```python
from build123d import *

# Parameters (mm, degrees)
SKETCH10_W         = 3
SKETCH10_H         = 3
HANDLE_DEPTH       = 8
SKETCH13_R         = 3
GUARD_DEPTH        = 1.5
SKETCH11_R         = 2
BLADE_DEPTH        = 25
BLADE_TAPER        = 1
BLADE_TIP_ANGLE    = 180
EASY_HAND_INSERT_R = 0.5
SCALE1_SCALE       = 2


with BuildPart() as part:
    # Sketch10 → Handle (new body)
    with BuildSketch(Plane(origin=(0, 0, 0), x_dir=(1, 0, 0), z_dir=(0, 1, 0))):
        Rectangle(SKETCH10_W, SKETCH10_H)
    extrude(amount=HANDLE_DEPTH)

    # Sketch13 → Guard (add)
    with BuildSketch(Plane(origin=(0, 8, 0), x_dir=(1, 0, 0), z_dir=(0, 1, 0))):
        with Locations(Location((0, 0, 0), (0, 0, 270))):
            Circle(SKETCH13_R)
    extrude(amount=GUARD_DEPTH)

    # Sketch11 → Blade (add)
    with BuildSketch(Plane(origin=(0, 9.5, 0), x_dir=(1, 0, 0), z_dir=(0, 1, 0))):
        Circle(SKETCH11_R)
    extrude(amount=BLADE_DEPTH, taper=BLADE_TAPER)

    # Sketch12 → Blade tip (revolve)
    with BuildSketch(Plane(origin=(0, 34.5, 0), x_dir=(1, 0, 0), z_dir=(0, 1, 0))):
        with BuildLine():
            Line((0, -1.563623377), (0, 1.563623377))
            ThreePointArc((0, 1.563623377), (-1.563623377, 0), (0, -1.563623377))
        make_face()
    revolve(axis=Axis((0, 34.5, 0), (0, 0, -1)), revolution_arc=BLADE_TIP_ANGLE)

    # Easy hand insert
    easy_hand_insert_edges = [part.edges().sort_by_distance(p)[0] for p in [
        (0, 0, 1.5),
        (-1.5, 0, 0),
        (0, 0, -1.5),
        (1.5, 0, 0),
        (1.5, 4, 1.5),
        (-1.5, 4, 1.5),
        (-1.5, 4, -1.5),
        (1.5, 4, -1.5),
    ]]
    fillet(easy_hand_insert_edges, radius=EASY_HAND_INSERT_R)


with BuildPart() as part_1:
    # Scale1: scaled about (0, 16.701239366, 0)
    add(part.part.scale(SCALE1_SCALE).moved(Location((0, -16.701239366, 0))))


solid = part_1.part
```
Check sheet for the modelled part. Datum: model origin and axes. Units: mm. A direction names the side the tool comes from. Round coordinates to 2 decimals unless told otherwise and drop trailing zeros. Order: outer loops, then holes, each group sorted by start corner. A loop starts at its lowest first (then second) coordinate and runs counter-clockwise, first axis right, second up. Notation, with made-up numbers: (63.5, 50) -> (112.5, 50) arc R25 ccw to (112.5, 65) -> close; hole circle Ø9 at (-1, 84). An arc over 180 degrees is marked (long way). Use CSV: the item, a comma, the result in double quotes.
(1) Cross-section at A-A (y = -8). Record the boundary of the cut face in (x, z), and give its area (3 significant figures).
Worked out:
outline,"(-3, -2) arc R1 ccw to (-2, -3) -> (2, -3) arc R1 ccw to (3, -2) -> (3, 2) arc R1 ccw to (2, 3) -> (-2, 3) arc R1 ccw to (-3, 2) -> close"
area,"35.1 mm²"
(2) Depth check by flat-ended pin: pin 1 (4.5 mm diameter, centred on y = -9.5, z = 1, fed in from -X); pin 2 (6 mm diameter, centred on x = 0, z = -4, fed in from +Y); pin 3 (4 mm diameter, centred on x = -4, y = 30, fed in from -Z). Enter the tip coordinate at first touch or a pass-through.
Worked out:
pin 1,"x = -3"
pin 2,"y = 55.26"
pin 3,"z = -2.89"
(3) Cross-section at C-C (y = 26.5). Record the boundary of the cut face in (x, z), and give its area (3 significant figures).
Worked out:
outline,"circle Ø7.16 at (0, 0)"
area,"40.2 mm²"
(4) Tool access check on faces 1 (the face through (-0.771, 27.649, 3.473)), 2 (the face through (-3, -8, 0)), 3 (the face through (0, -8, -3)). Record the directions out of +Z, -Z, +X, -X, +Y, -Y that give a thin tool (end or side, any length) a straight path to the whole face; none if there is none.
Worked out:
face 1,"+Y"
face 2,"+Z, -Z, -X, -Y"
face 3,"-Z, +X, -X, -Y"
(5) Cross-section at B-B (y = 49). Record the boundary of the cut face in (x, z).
Worked out:
outline,"circle Ø6.37 at (0, 0)"
(6) Material ranges on line 1 along X through (y, z) = (-8, 0.25); line 2 along Y through (x, z) = (-0.75, -5), recorded low to high. Write a range as from..to.
Worked out:
line 1,"-3..3"
line 2,"-0.7..2.3"
